```python
from build123d import *

# Parameters (mm, degrees)
SCHIZZO1_R                  = 115
ESTRUSIONE1_DEPTH           = 6
SCHIZZO2_W                  = 30
SCHIZZO2_H                  = 46
ESTRUSIONE2_DEPTH           = 10
RIPETIZIONECIRCOLARE1_COUNT = 8
SCHIZZO4_R                  = 30
ESTRUSIONE3_DEPTH           = 163.941707368
SCHIZZO5_R                  = 5
ESTRUSIONE4_DEPTH           = 163.941707368


with BuildPart() as part:
    # Schizzo1 → Estrusione1 (new body)
    with BuildSketch(Plane.XY):
        Circle(SCHIZZO1_R)
    extrude(amount=ESTRUSIONE1_DEPTH)

    # Schizzo2 → Estrusione2 (add)
    with BuildSketch(Plane.XY.offset(6)):
        with Locations((0, 91.01754251)):
            Rectangle(SCHIZZO2_W, SCHIZZO2_H)
    estrusione2 = extrude(amount=ESTRUSIONE2_DEPTH)

    # RipetizioneCircolare1: Estrusione2 ×8 about axis
    ripetizionecircolare1_axis = Axis((0, 0, 6), (0, 0, -1))
    for i in range(1, RIPETIZIONECIRCOLARE1_COUNT):
        add(estrusione2.rotate(ripetizionecircolare1_axis, i * 360 / RIPETIZIONECIRCOLARE1_COUNT))

    # Schizzo4 → Estrusione3 (cut, through all)
    with BuildSketch(Plane.XY.offset(6)):
        Circle(SCHIZZO4_R)
    extrude(amount=-ESTRUSIONE3_DEPTH, mode=Mode.SUBTRACT)

    # Schizzo5 → Estrusione4 (cut, through all)
    with BuildSketch(Plane.XY.offset(6)):
        with Locations((0, 40)):
            Circle(SCHIZZO5_R)
    extrude(amount=-ESTRUSIONE4_DEPTH, mode=Mode.SUBTRACT)


solid = part.part
```
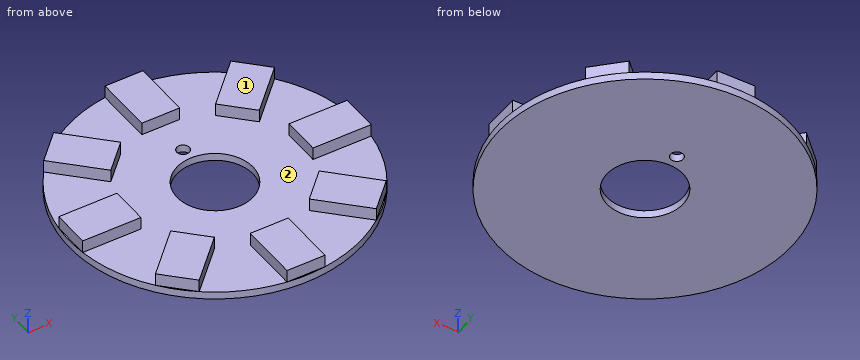
Source: CAD feature listing. Evaluate the final solid. Frame: model axes, mm. Face numbers are marked on the shaded views. Coordinates: 2 decimals unless noted, no trailing zeros. Write each loop counter-clockwise with the first axis right and the second up, starting at its lowest first coordinate (ties: lowest second). Pieces come first, ordered by that corner, then holes. Notation, with made-up numbers: (65.25, 21) -> (100.25, 21) arc R17 ccw to (100.25, 52) -> close; hole circle Ø1 at (6, 84.5). An arc over 180 degrees is marked (long way). Return JSON: item names as keys, results as strings. Group by question number.
1) Section query A-A, the plane y = 0. Return loops of the section in (x, z).
2) Section query B-B, the plane z = 10.5. State how many separate pieces and enclosed holes the cut face has, plus the area to 3 significant figures.
3) Contact query for flat-ended pins moving along their axis: P1, Ø3, axis at x = 43, y = 76, coming from the +Z side; P2, Ø3, axis at y = 7, z = 11, coming from the -X side; P3, Ø4, axis at y = -48, z = 12.5, coming from the -X side. Output: stop coordinate, or through.
4) Mould query, pull axis X, two halves, no side actions, for the marked faces 1 and 2. Classes: +X half, -X half, draft (parallel to the pull), parting line (faces both ways), or undercut.
5) Ray query, line 1 along Y through (x, z) = (0, 4.2); line 2 along Y through (x, z) = (-1.5, 1); line 3 along X through (y, z) = (-98, 8.75). Return the intervals inside material, ascending.
6) Section query C-C, the plane x = 0. Return loops of the section in (y, z), plus the area to 3 significant figures.
7) Section query D-D, the plane y = 101. Return loops of the section in (x, z), plus the area to 3 significant figures.
From the geometry:
{
 "1": {"outline": "(-115, 0) -> (-30, 0) -> (-30, 6) -> (-68.02, 6) -> (-68.02, 16) -> (-114.02, 16) -> (-114.02, 6) -> (-115, 6) -> close; (30, 0) -> (115, 0) -> (115, 6) -> (114.02, 6) -> (114.02, 16) -> (68.02, 16) -> (68.02, 6) -> (30, 6) -> close"},
 "2": {"separate pieces": "8", "enclosed holes": "0", "area": "11,000 mm²"},
 "3": {"P1": "z = 6", "P2": "x = -114.02", "P3": "x = -71.21"},
 "4": {"face 1": "draft", "face 2": "undercut"},
 "5": {"line 1": "-115 to -30, 30 to 35, 45 to 115", "line 2": "-114.99 to -29.96, 29.96 to 35.23, 44.77 to 114.99", "line 3": "-15 to 15"},
 "6": {"outline": "(-115, 0) -> (-30, 0) -> (-30, 6) -> (-68.02, 6) -> (-68.02, 16) -> (-114.02, 16) -> (-114.02, 6) -> (-115, 6) -> close; (30, 0) -> (35, 0) -> (35, 6) -> (30, 6) -> close; (45, 0) -> (115, 0) -> (115, 6) -> (114.02, 6) -> (114.02, 16) -> (68.02, 16) -> (68.02, 6) -> (45, 6) -> close", "area": "1,880 mm²"},
 "7": {"outline": "(-54.99, 0) -> (54.99, 0) -> (54.99, 6) -> (15, 6) -> (15, 16) -> (-15, 16) -> (-15, 6) -> (-54.99, 6) -> close", "area": "960 mm²"}
}
